```python
from build123d import *

# Parameters (mm, degrees)
SKETCH1_R                               = 15
BOSS_EXTRUDE1_DEPTH                     = 3.5
SKETCH2_R                               = 3.9
CUT_EXTRUDE1_DEPTH                      = 22.5
CBORE_FOR_M5_HEX_HEAD_BOLT1_D           = 2.5
CBORE_FOR_M5_HEX_HEAD_BOLT1_CBORE_D     = 5.5
CBORE_FOR_M5_HEX_HEAD_BOLT1_CBORE_DEPTH = 2.5
TAP_DRILL_FOR_M3X0_5_TAP1_D             = 2.7
SKETCH9_R                               = 2.35
SKETCH9_R_2                             = 1.35
BOSS_EXTRUDE2_DEPTH                     = 1


with BuildPart() as part:
    # Sketch1 → Boss-Extrude1 (new body)
    with BuildSketch(Plane(origin=(0, 0, 0), x_dir=(1, 0, 0), z_dir=(0, 1, 0))):
        with Locations(Location((0, 0, 0), (0, 0, 90))):
            Circle(SKETCH1_R)
    extrude(amount=BOSS_EXTRUDE1_DEPTH)

    # Sketch2 → Cut-Extrude1 (cut, through all)
    with BuildSketch(Plane(origin=(0, 3.5, 0), x_dir=(1, 0, 0), z_dir=(0, 1, 0))):
        with Locations(Location((0, 0, 0), (0, 0, 270))):
            Circle(SKETCH2_R)
    extrude(amount=-CUT_EXTRUDE1_DEPTH, mode=Mode.SUBTRACT)

    # CBORE for M5 Hex Head Bolt1 (through all)
    with Locations(Plane(origin=(0, 3.5, 0), x_dir=(1, 0, 0), z_dir=(0, 1, 0))):
        with Locations((-6, 0), (0, 6), (6, 0), (0, -6)):
            CounterBoreHole(CBORE_FOR_M5_HEX_HEAD_BOLT1_D / 2, CBORE_FOR_M5_HEX_HEAD_BOLT1_CBORE_D / 2, CBORE_FOR_M5_HEX_HEAD_BOLT1_CBORE_DEPTH)

    # Tap Drill for M3x0.5 Tap1 (through all)
    with Locations(Plane(origin=(0, 3.5, 0), x_dir=(1, 0, 0), z_dir=(0, 1, 0))):
        with Locations((-8, 8), (8, 8), (8, -8), (-8, -8)):
            Hole(TAP_DRILL_FOR_M3X0_5_TAP1_D / 2)

    # Sketch9 → Boss-Extrude2 (add)
    # profile 1 of 4: a face of its own
    with BuildSketch(Plane(origin=(0, 3.5, 0), x_dir=(1, 0, 0), z_dir=(0, 1, 0))):
        with Locations(Location((8, -8, 0), (0, 0, 270))):
            Circle(SKETCH9_R)
        with Locations(Location((8, -8, 0), (0, 0, 270))):
            Circle(SKETCH9_R_2, mode=Mode.SUBTRACT)
    # profile 2 of 4: a face of its own
    with BuildSketch(Plane(origin=(0, 3.5, 0), x_dir=(1, 0, 0), z_dir=(0, 1, 0))):
        with Locations(Location((8, 8, 0), (0, 0, 270))):
            Circle(SKETCH9_R)
        with Locations(Location((8, 8, 0), (0, 0, 270))):
            Circle(SKETCH9_R_2, mode=Mode.SUBTRACT)
    # profile 3 of 4: a face of its own
    with BuildSketch(Plane(origin=(0, 3.5, 0), x_dir=(1, 0, 0), z_dir=(0, 1, 0))):
        with Locations(Location((-8, -8, 0), (0, 0, 270))):
            Circle(SKETCH9_R)
        with Locations(Location((-8, -8, 0), (0, 0, 270))):
            Circle(SKETCH9_R_2, mode=Mode.SUBTRACT)
    # profile 4 of 4: a face of its own
    with BuildSketch(Plane(origin=(0, 3.5, 0), x_dir=(1, 0, 0), z_dir=(0, 1, 0))):
        with Locations(Location((-8, 8, 0), (0, 0, 270))):
            Circle(SKETCH9_R)
        with Locations(Location((-8, 8, 0), (0, 0, 270))):
            Circle(SKETCH9_R_2, mode=Mode.SUBTRACT)
    extrude(amount=BOSS_EXTRUDE2_DEPTH)


solid = part.part
```
Model file for the job. Use its own axes, mm. A direction names the side the tool comes from. Coordinates: 2 decimals unless noted, no trailing zeros. Loops run counter-clockwise (first coordinate to the right, second up) from the corner with the lowest first, then second, coordinate; pieces in that order, holes last. Notation, with made-up numbers: (16, 80.25) - (27, 80.25) arc R28 ccw to (27, 115.25) - close; hole circle Ø6 at (30, 87.5). An arc over 180 degrees is marked (long way). Answer as a JSON object with one key per item and string values. Group by question number.
(1) Flat gauge pins, fed straight in: pin 1 (2 mm diameter, centred on x = 6, z = 0, fed in from +Y); pin 2 (1.5 mm diameter, centred on y = 1.5, z = -3.5, fed in from -X); pin 3 (4.5 mm diameter, centred on x = 0, z = 6, fed in from +Y); pin 4 (4 mm diameter, centred on x = 3.5, z = -2.5, fed in from +Y). Where does each tip first touch, or does it go through?
(2) Probe line 1 along X through (y, z) = (4, 8); line 2 along Z through (x, y) = (-7.25, 1.5); line 3 along X through (y, z) = (1.85, -8). List the from-to ranges inside material, lowest first.
(3) Cut at D-D (z = -6). Give the cut face in (x, y), then the cut area to 3 significant figures.
(4) Cut at A-A (x = 0). Give the cut face in (y, z), then the cut area to 4 significant figures.
(5) Tool access for faces 1 (the face through (6, 4.5, 8)), 2 (the face through (0, 1, -7.4)): list every direction of +Z, -Z, +X, -X, +Y, -Y with a clear straight run to the whole face (end or side of a thin tool).
(6) Cut at C-C (x = -6). Give the cut face in (y, z), then the cut area to 3 significant figures.
(7) Cut at B-B (z = 0). Give the cut face in (x, y), then the cut area to 4 significant figures.
(8) Two-plate mould, pull along Z, no slides. Class faces 3 (the face through (0.27, 0.49, -4.78)), 4 (the face through (-0.66, 1.726, 14.985)), 5 (the face through (6, 4.5, -8)): released by +Z, released by -Z, zero draft, split by the parting line, or undercut.
Geometry says:
{
 "1": {"pin 1": "passes through", "pin 2": "stops at x = -14.75", "pin 3": "stops at y = 1", "pin 4": "stops at y = 3.5"},
 "2": {"line 1": "x = -10.35 to -9.35, -6.65 to -5.65, 5.65 to 6.65, 9.35 to 10.35", "line 2": "z = -13.13 to -9.12, -6.88 to -2.45, 2.45 to 6.88, 9.12 to 13.13", "line 3": "x = -12.69 to -9.35, -6.65 to -1.89, 1.89 to 6.65, 9.35 to 12.69"},
 "3": {"outline": "(-13.75, 0) - (-1.25, 0) - (-1.25, 1) - (-2.75, 1) - (-2.75, 3.5) - (-6.77, 3.5) - (-6.77, 4.5) - (-9.23, 4.5) - (-9.23, 3.5) - (-13.75, 3.5) - close; (1.25, 0) - (13.75, 0) - (13.75, 3.5) - (9.23, 3.5) - (9.23, 4.5) - (6.77, 4.5) - (6.77, 3.5) - (2.75, 3.5) - (2.75, 1) - (1.25, 1) - close", "area": "84.9 mm^2"},
 "4": {"outline": "(0, -15) - (3.5, -15) - (3.5, -8.75) - (1, -8.75) - (1, -7.25) - (0, -7.25) - close; (0, -4.75) - (1, -4.75) - (1, -3.9) - (0, -3.9) - close; (0, 3.9) - (1, 3.9) - (1, 4.75) - (0, 4.75) - close; (0, 7.25) - (1, 7.25) - (1, 8.75) - (3.5, 8.75) - (3.5, 15) - (0, 15) - close", "area": "48.45 mm^2"},
 "5": {"face 1": "+Z, -Z, +X, -X, +Y", "face 2": "+Y"},
 "6": {"outline": "(0, -13.75) - (3.5, -13.75) - (3.5, -9.23) - (4.5, -9.23) - (4.5, -6.77) - (3.5, -6.77) - (3.5, -2.75) - (1, -2.75) - (1, -1.25) - (0, -1.25) - close; (0, 1.25) - (1, 1.25) - (1, 2.75) - (3.5, 2.75) - (3.5, 6.77) - (4.5, 6.77) - (4.5, 9.23) - (3.5, 9.23) - (3.5, 13.75) - (0, 13.75) - close", "area": "84.9 mm^2"},
 "7": {"outline": "(-15, 0) - (-7.25, 0) - (-7.25, 1) - (-8.75, 1) - (-8.75, 3.5) - (-15, 3.5) - close; (-4.75, 0) - (-3.9, 0) - (-3.9, 1) - (-4.75, 1) - close; (3.9, 0) - (4.75, 0) - (4.75, 1) - (3.9, 1) - close; (7.25, 0) - (15, 0) - (15, 3.5) - (8.75, 3.5) - (8.75, 1) - (7.25, 1) - close", "area": "48.45 mm^2"},
 "8": {"face 3": "undercut", "face 4": "split by the parting line", "face 5": "zero draft"}
}
